Can you work these out from the model? Positions are in its coordinate system, mm. A direction names the side the tool comes from. Coordinates: 2 decimals unless noted, no trailing zeros. Loops run counter-clockwise (first coordinate to the right, second up) from the corner with the lowest first, then second, coordinate; pieces in that order, holes last. Notation, with made-up numbers: (-20, 51) -> (-3, 51) arc R30 cw to (-3, 76) -> close; hole circle Ø8 at (48.25, 34). An arc over 180 degrees is marked (long way). Put each result on its own line as item: value. Start each with the question number.
Item 1: If we section it at B-B on x = 9: Please give me the cut outline in (y, z).
Item 2: Will these pins go through, and if not, where does the flat tip stop? P1, Ø3, axis at y = -20.5, z = 1, coming from the -X side; P2, Ø8, axis at x = 10.5, z = 5, coming from the -Y side; P3, Ø5, axis at y = -6, z = 0, coming from the +X side.
Item 3: If we section it at D-D on z = -4.5: Please give me the cut outline in (x, y), plus the area to 3 significant figures.
Item 4: If we section it at A-A on y = -21: Please give me the cut outline in (x, z).
Item 5: Please list where these lines run through material, in increasing order: L1, parallel to Y at x = -14.5, z = 0; L2, parallel to Z at x = 10, y = 3; L3, parallel to X at y = -9.5, z = 2.75. Write a range as from..to.
Item 6: We'd pull the mould along Z, two halves only. Please class faces 4 (the flat face through (-6, 1, -10)), 5 (the flat face through (12.01, 5.07, -3.12)), 6 (the flat face through (11.956, 5.07, 3.209)), 7 (the flat face through (-17.5, -9, 0)): pulls with the +Z half, pulls with the -Z half, needs draft (parallel to the pull), parting line crosses it, or undercut.
Item 7: For faces 1 (the flat face through (17.5, 5, 0)), 2 (the flat face through (1.044, 5.07, -3.209)), 3 (the flat face through (-1, 0, 0)), which set-ups out of +Z, -Z, +X, -X, +Y, -Y let a thin tool reach every point of the face, with its end or its side?
Item 8: If we section it at C-C on y = 2: Please give me the cut outline in (x, z).
```python
from build123d import *

# Parameters (mm, degrees)
SKETCH1_W           = 35
SKETCH1_H           = 20
BOSS_EXTRUDE1_DEPTH = 10
FILLET1_R           = 5
CUT_EXTRUDE2_DEPTH  = 23.5
SKETCH5_W           = 4.5
SKETCH5_H           = 20
BOSS_EXTRUDE3_DEPTH = 28
SKETCH6_R           = 1.85
CUT_EXTRUDE3_DEPTH  = 43.594013664


with BuildPart() as part:
    # Sketch1 → Boss-Extrude1 (new body)
    with BuildSketch(Plane(origin=(0, 0, 0), x_dir=(1, 0, 0), z_dir=(0, 1, 0))):
        Rectangle(SKETCH1_W, SKETCH1_H)
    extrude(amount=BOSS_EXTRUDE1_DEPTH)

    # Fillet1
    fillet1_edges = [part.edges().sort_by_distance(p)[0] for p in [
        (17.5, 5, 10),
        (17.5, 5, -10),
    ]]
    fillet(fillet1_edges, radius=FILLET1_R)

    # Sketch4 → Cut-Extrude2 (cut, through all)
    with BuildSketch(Plane(origin=(0, 10, 0), x_dir=(1, 0, 0), z_dir=(0, 1, 0))):
        Polygon((10.154627204, -6.33), (13.809254408, 0), (10.154627204, 6.33), (2.845372796, 6.33), (-0.809254408, 0), (2.845372796, -6.33), align=None)
    extrude(amount=-CUT_EXTRUDE2_DEPTH, mode=Mode.SUBTRACT)

    # Sketch5 → Boss-Extrude3 (add)
    with BuildSketch(Plane.XZ):
        with Locations((-15.25, 0)):
            Rectangle(SKETCH5_W, SKETCH5_H)
    extrude(amount=BOSS_EXTRUDE3_DEPTH)

    # Sketch6 → Cut-Extrude3 (cut, through all)
    with BuildSketch(Plane(origin=(-13, 0, 0), x_dir=(0, 0, -1), z_dir=(1, 0, 0))):
        with Locations((0, -6)):
            Circle(SKETCH6_R)
        with Locations((0, -21)):
            Circle(SKETCH6_R)
    extrude(amount=-CUT_EXTRUDE3_DEPTH, mode=Mode.SUBTRACT)


solid = part.part
```
Solutions:
1. outline: (0, -10) -> (10, -10) -> (10, -6.33) -> (0, -6.33) -> close; (0, 6.33) -> (10, 6.33) -> (10, 10) -> (0, 10) -> close
2. P1: x = -17.5
2. P2: y = 0
2. P3: x = -13
3. outline: (-17.5, -28) -> (-13, -28) -> (-13, 0) -> (1.79, 0) -> (1.79, 10) -> (-17.5, 10) -> close; (11.21, 0) -> (17.5, 0) -> (17.5, 10) -> (11.21, 10) -> close
3. area: 382 mm^2
4. outline: (-17.5, -10) -> (-13, -10) -> (-13, -1.85) -> (-17.5, -1.85) -> close; (-17.5, 1.85) -> (-13, 1.85) -> (-13, 10) -> (-17.5, 10) -> close
5. L1: -28..-22.85, -19.15..-7.85, -4.15..10
5. L2: -10..-6.33, 6.33..10
5. L3: -17.5..-13
6. face 4: pulls with the -Z half
6. face 5: undercut
6. face 6: undercut
6. face 7: needs draft
7. face 1: +Z, -Z, +X, +Y, -Y
7. face 2: +Y, -Y
7. face 3: +Z, -Z, +X, -Y
8. outline: (-17.5, -10) -> (12.5, -10) arc R5 ccw to (17.5, -5) -> (17.5, 5) arc R5 ccw to (12.5, 10) -> (-17.5, 10) -> close; hole (-0.81, 0) -> (2.85, -6.33) -> (10.15, -6.33) -> (13.81, 0) -> (10.15, 6.33) -> (2.85, 6.33) -> close
